Source: CAD feature listing. Evaluate the final solid. Frame: model axes, mm. A direction names the side the tool comes from. Coordinates: 2 decimals unless noted, no trailing zeros. Loops run counter-clockwise (first coordinate to the right, second up) from the corner with the lowest first, then second, coordinate; pieces in that order, holes last.
Item 1: Line query: probe 1 along Z at (x, y) = (-22, 0.55); probe 2 along Z at (x, y) = (20.5, 0.8); probe 3 along Z at (x, y) = (-24.5, 0.25). Output: solid intervals per line, ascending.
Item 2: Section query A-A, the plane y = 1.75. Return the cut outline in (x, z) (3 decimals), then the cut area to 3 significant figures.
Item 3: Section query B-B, the plane z = 6.06. Return the cut outline in (x, y) (3 decimals).
Item 4: Pull-direction query (Z, two-part tool) for faces 3 (the cylindrical face through (-25.6, 1.48, -0.43)), 4 (the cylindrical face through (-27.643, 1.479, -0.113)), 5 (the flat face through (17.373, 1.479, 1.695)); classes: +Z half, -Z half, draft (parallel to the pull), parting line (faces both ways), or undercut.
Item 5: Section query C-C, the plane x = 11. Return the cut outline in (y, z), then the cut area to 3 significant figures.
Item 6: Reachability of faces 1 (the flat face through (-8.94, 1.48, 1.06)), 2 (the flat face through (-1, 0, -1)) from +Z, -Z, +X, -X, +Y, -Y: full face, straight path, thin tool, end or side. Return the list, or none.
```python
from build123d import *

# Parameters (mm, degrees)
SKETCH1_R           = 2
BOSS_EXTRUDE1_DEPTH = 3


with BuildPart() as part:
    # Sketch1 → Boss-Extrude1 (new body)
    with BuildSketch(Plane(origin=(0, 0, 0), x_dir=(-1, 0, 0), z_dir=(0, 1, 0))):
        with BuildLine():
            Line((-13.023955953, -3.551475079), (23.596044053, -3.999700403))
            ThreePointArc((23.596044053, -3.999700403), (27.6449251, -0.024478432), (23.645, 4))
            Line((23.645, 4), (-6.179618863, -1.958864922))
            ThreePointArc((-6.179618863, -1.958864922), (-7.859851478, -1.510674898), (-8.52802301, 0.094816535))
            ThreePointArc((-8.52802301, 0.094816535), (-9.929506285, 1.686957231), (-11.521937407, 0.285803961))
            ThreePointArc((-11.521937407, 0.285803961), (-12.027681304, -0.523458534), (-12.981727074, -0.545352487))
            Line((-12.981727074, -0.545352487), (-21.889675517, 3.998669315))
            ThreePointArc((-21.889675517, 3.998669315), (-22.389088805, 4.58847924), (-22.319318125, 5.358168419))
            ThreePointArc((-22.319318125, 5.358168419), (-22.943168419, 7.385681875), (-24.970681875, 6.761831581))
            ThreePointArc((-24.970681875, 6.761831581), (-25.256630844, 3.706810464), (-23.29448222, 1.347807789))
            Line((-23.29448222, 1.347807789), (-14.834203373, -3.093435701))
            ThreePointArc((-14.834203373, -3.093435701), (-13.956181951, -3.429568117), (-13.023955953, -3.551475079))
        make_face()
        with Locations(Location((23.645, 0, 0), (0, 0, 90))):
            Circle(SKETCH1_R, mode=Mode.SUBTRACT)
    extrude(amount=BOSS_EXTRUDE1_DEPTH)


solid = part.part
```
Verdict:
1. probe 1: z = -3.98 to -1.14, 1.14 to 3.67
1. probe 2: z = -0.12 to 3.29
1. probe 3: z = -3.91 to -1.81, 1.81 to 3.91
2. outline: (-23.645, 4) arc R4 ccw (long way) to (-23.596, -4) - (13.024, -3.551) arc R4 ccw to (14.834, -3.093) - (23.294, 1.348) arc R4.001 ccw to (24.971, 6.762) arc R1.5 ccw to (22.319, 5.358) arc R1.001 cw to (21.89, 3.999) - (12.982, -0.545) arc R1.005 cw to (11.522, 0.286) arc R1.5 ccw to (8.528, 0.095) arc R1.967 cw to (6.18, -1.959) - close; hole circle Ø4 at (-23.645, 0)
2. area: 229 mm2
3. outline: (22.145, 0) - (25.261, 0) - (25.261, 3) - (22.145, 3) - close
4. face 3: undercut
4. face 4: parting line
4. face 5: +Z half
5. outline: (0, -3.58) - (3, -3.58) - (3, 1.33) - (0, 1.33) - close
5. area: 14.7 mm2
6. face 1: +Z, +Y, -Y
6. face 2: +Z, -Z, +X, -X, -Y
